Build history of the part. All positions in model axes, mm. A direction names the side the tool comes from. Coordinates: 2 decimals unless noted, no trailing zeros. Order: outer loops, then holes, each group sorted by start corner. A loop starts at its lowest first (then second) coordinate and runs counter-clockwise, first axis right, second up. Notation, with made-up numbers: (34.25, 27) - (41.25, 27) arc R17 cw to (41.25, 36) - close; hole circle Ø8 at (62, 85.5). An arc over 180 degrees is marked (long way). Return JSON: item names as keys, results as strings.
from build123d import *

# Parameters (mm, degrees)
PAD_DEPTH = 14.8


with BuildPart() as part:
    # Sketch → Pad (new body)
    with BuildSketch(Plane.XY):
        with BuildLine():
            Line((0, 89.13), (14.815, 89.13))
            ThreePointArc((17.289752, 86.275597), (16.703916, 88.26768), (14.815, 89.13))
            Line((17.289752, 86.275597), (9.699752, 33.275597))
            ThreePointArc((7.225, 31.13), (8.86268, 31.741084), (9.699752, 33.275597))
            Line((7.225, 31.13), (0, 31.13))
            Line((0, 31.13), (0, 0))
            Line((9.315394, 0), (0, 0))
            ThreePointArc((9.315394, 0), (29.707786, 7.609217), (40.131008, 26.716971))
            Line((48.437046, 84.716971), (40.131008, 26.716971))
            ThreePointArc((48.437046, 84.716971), (41.142215, 109.522392), (17.621432, 120.26))
            Line((0, 120.26), (17.621432, 120.26))
            Line((0, 120.26), (0, 89.13))
        make_face()
    pad = extrude(amount=PAD_DEPTH)

    # Mirrored: Pad across Sketch V_Axis
    add(pad.mirror(Plane(origin=(0, 0, 0), x_dir=(0, 0, 1), z_dir=(1, 0, 0))))


solid = part.part
1. Probe L1, parallel to Y at x = 7, z = 3; L2, parallel to X at y = 59, z = 7.75; L3, parallel to X at y = 81, z = 8. List the from-to ranges inside material, lowest first.
Check values:
{"L1": "0 to 31.13, 89.13 to 120.26", "L2": "-44.75 to -13.38, 13.38 to 44.75", "L3": "-47.9 to -16.53, 16.53 to 47.9"}
2. Drop flat-ended pins along their axis: pin 1 (12 mm diameter, centred on x = 18.5, y = 36, fed in from -Z); pin 2 (4 mm diameter, centred on x = -21, z = 3.5, fed in from +Y); pin 3 (5 mm diameter, centred on y = 98, z = 6, fed in from +X); pin 4 (2 mm diameter, centred on y = 16, z = 7.5, fed in from -X). Give the stop position or say it passes through.
Check values:
{"pin 1": "z = 0", "pin 2": "y = 120.23", "pin 3": "x = 48.09", "pin 4": "x = -37.05"}
3. Tool access for faces 4 (the cylindrical face through (-29.472, 7.406, 7.296)), 5 (the flat face through (13.55, 60.15, 7.3)): list every direction of +Z, -Z, +X, -X, +Y, -Y with a clear straight run to the whole face (end or side of a thin tool).
Check values:
{"face 4": "+Z, -Z, -X, -Y", "face 5": "+Z, -Z"}
4. Cut at C-C on y = 37.5. Give the cut face in (x, z).
Check values:
{"outline": "(-41.68, 0) - (-10.3, 0) - (-10.3, 14.8) - (-41.68, 14.8) - close; (10.3, 0) - (41.68, 0) - (41.68, 14.8) - (10.3, 14.8) - close"}
5. Cut at A-A on z = 4.75. Give the cut face in (x, y) (3 decimals), plus the area to 3 significant figures.
Check values:
{"outline": "(-48.437, 84.717) - (-40.131, 26.717) arc R31.13 ccw to (-9.315, 0) - (9.315, 0) arc R31.13 ccw to (40.131, 26.717) - (48.437, 84.717) arc R31.13 ccw to (17.621, 120.26) - (-17.621, 120.26) arc R31.13 ccw to start; hole (-17.29, 86.276) - (-9.7, 33.276) arc R2.5 ccw to (-7.225, 31.13) - (7.225, 31.13) arc R2.5 ccw to (9.7, 33.276) - (17.29, 86.276) arc R2.5 ccw to (14.815, 89.13) - (-14.815, 89.13) arc R2.5 ccw to start", "area": "8,370 mm²"}
6. Cut at D-D on x = -37. Give the cut face in (y, z).
Check values:
{"outline": "(16.89, 0) - (113.49, 0) - (113.49, 14.8) - (16.89, 14.8) - close"}
7. Mould opens along X. For faces 1 (the flat face through (-44.34, 56.12, 7.3)), 2 (the cylindrical face through (16.723, 88.245, 7.296)), 3 (the flat face through (0, 0, 7)) say: pulls with the +X half, pulls with the -X half, needs draft (parallel to the pull), parting line crosses it, or undercut.
Check values:
{"face 1": "pulls with the -X half", "face 2": "undercut", "face 3": "needs draft"}
8. Cut at B-B on x = 2.5. Give the cut face in (y, z).
Check values:
{"outline": "(0, 0) - (31.13, 0) - (31.13, 14.8) - (0, 14.8) - close; (89.13, 0) - (120.26, 0) - (120.26, 14.8) - (89.13, 14.8) - close"}
